Answer from the drawing. Dimensions are ordinates in mm from the lowest x, y and z of the part. Give positions to 0.01 mm unless a question says otherwise; leave off trailing zeros. Write each loop counter-clockwise with the first axis right and the second up, starting at its lowest first coordinate (ties: lowest second). Pieces come first, ordered by that corner, then holes. Notation, with made-up numbers: (-39.5, 18) -> (-29.5, 18) arc R17 cw to (-29.5, 50) -> close; hole circle Ø5 at (5, -35). An arc over 180 degrees is marked (long way). Use a Markdown table: item, result. Add a question column.
Q1. Each of these flat-tipped pins is pushed along its axis until it touches: pin 1 Ø1.2 at (x, z) = (61.5, 3) entering from -Y; pin 2 Ø2 at (y, z) = (8, 2.5) entering from +X; pin 3 Ø2 at (x, z) = (66.5, 1.5) entering from +Y; pin 4 Ø4 at (x, y) = (20, 35) entering from -Z. Where does it stop, or does it pass through?
Q2. Section C-C, the plane y = 7 is taken. Give the vertices of the cut face in (x, z), plus the area to 3 significant figures.
Q3. Section B-B, the plane x = 80 is taken. Give the vertices of the cut face in (y, z), plus the area to 3 significant figures.
Q4. Section D-D, the plane x = 5 is taken. Give the vertices of the cut face in (y, z).
Q5. Consider line 1 (Y direction, x = 80, z = 2.8); line 2 (Y direction, x = 15, z = 1.75); line 3 (Y direction, x = 13.5, z = 1.55). Determine where each line is inside the solid, lowest interval first.
Q6. Section A-A, the plane y = 35 is taken. Give the vertices of the cut face in (x, z), plus the area to 3 significant figures.
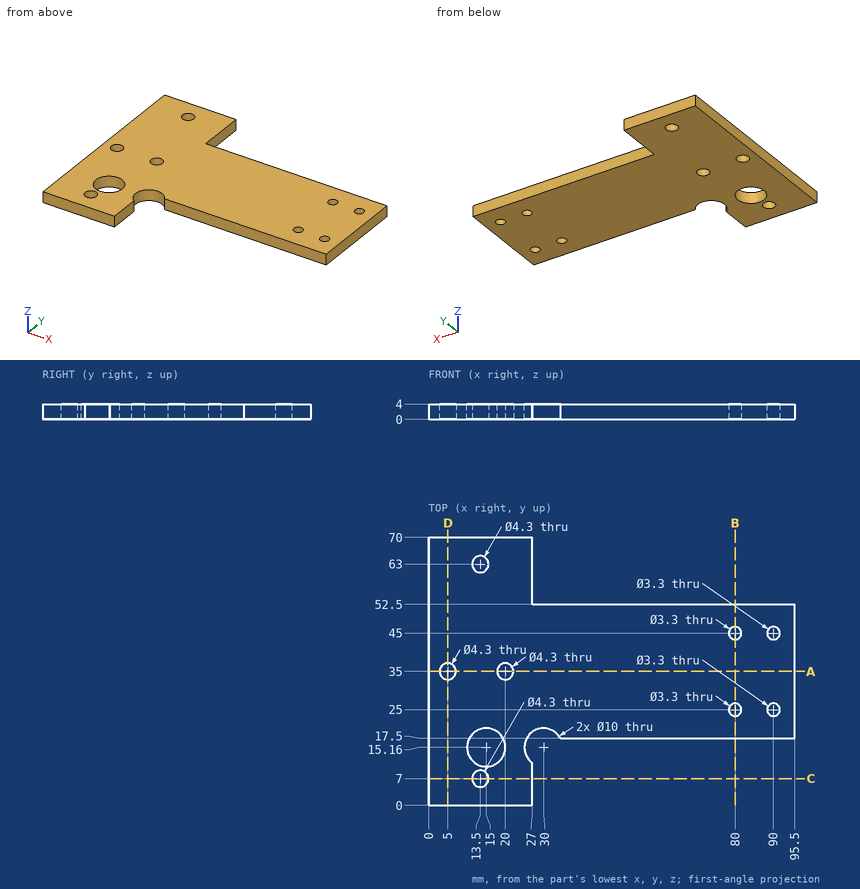
Result set:
| question | item | result |
|---|---|---|
| 1 | pin 1 | stops at y = 17.5 |
| 1 | pin 2 | stops at x = 27 |
| 1 | pin 3 | stops at y = 52.5 |
| 1 | pin 4 | passes through |
| 2 | outline | (0, 0) -> (11.35, 0) -> (11.35, 4) -> (0, 4) -> close; (15.65, 0) -> (27, 0) -> (27, 4) -> (15.65, 4) -> close |
| 2 | area | 90.8 mm2 |
| 3 | outline | (17.5, 0) -> (23.35, 0) -> (23.35, 4) -> (17.5, 4) -> close; (26.65, 0) -> (43.35, 0) -> (43.35, 4) -> (26.65, 4) -> close; (46.65, 0) -> (52.5, 0) -> (52.5, 4) -> (46.65, 4) -> close |
| 3 | area | 114 mm2 |
| 4 | outline | (0, 0) -> (32.85, 0) -> (32.85, 4) -> (0, 4) -> close; (37.15, 0) -> (70, 0) -> (70, 4) -> (37.15, 4) -> close |
| 5 | line 1 | y = 17.5 to 23.35, 26.65 to 43.35, 46.65 to 52.5 |
| 5 | line 2 | y = 0 to 5.46, 8.54 to 10.16, 20.16 to 61.46, 64.54 to 70 |
| 5 | line 3 | y = 0 to 4.85, 9.15 to 10.39, 19.93 to 60.85, 65.15 to 70 |
| 6 | outline | (0, 0) -> (2.85, 0) -> (2.85, 4) -> (0, 4) -> close; (7.15, 0) -> (17.85, 0) -> (17.85, 4) -> (7.15, 4) -> close; (22.15, 0) -> (95.5, 0) -> (95.5, 4) -> (22.15, 4) -> close |
| 6 | area | 348 mm2 |
